Can you work these out from the model? Positions are in its coordinate system, mm. A direction names the side the tool comes from. Coordinates: 2 decimals unless noted, no trailing zeros. Order: outer loops, then holes, each group sorted by start corner. A loop starts at its lowest first (then second) coordinate and runs counter-clockwise, first axis right, second up. Notation, with made-up numbers: M 68.5,20 L 107.5,20 A8 cw 107.5,24 Z; hole C 69.5,79.25 d2. An arc over 180 degrees is marked long. Answer as CSV lines item,"result". Start each with the question number.
1. Will this pin go through, and if not, where does the flat tip stop? pin 1 (10 mm diameter, centred on x = 41, y = -49.5, fed in from -Z).
2. If we mould it in two halves opening along X, with no side actions, what happens to faces 3 (the face through (25, -61, 1.4)), 4 (the face through (-104.866, -60.837, 1.226)), 5 (the face through (-100.82, 56.74, 0.2)), 6 (the face through (100.82, -56.74, 0.2))? For each: released by +X, released by -X, zero draft, split by the parting line, or undercut.
3. I need wall thicknesses on line 1 along X through (y, z) = (-3, 0.4); line 2 along Y through (x, z) = (47.5, 0.45); line 3 along Y through (x, z) = (-3.5, 0.35). Which ranges of each line are inside material? Lowest first, please. Write a range as from..to.
4. If we section it at B-B (x = 53): List the corners of the cut face in (y, z) for me, plus the area to 3 significant figures.
5. On a 3-axis mill with a long thin cutter (end or side, diameter ignored), from which of +Z, -Z, +X, -X, +Y, -Y can I reach the whole of each face in a straight line? I mean faces 1 (the face through (-100.94, -56.62, 0.2)), 2 (the face through (-105.037, 60.666, 1.226)). Say none if no direction works.
6. If we section it at C-C (z = 0.65): List the corners of the cut face in (x, y) for me.
7. If we section it at A-A (y = -3.5): List the corners of the cut face in (x, z) for me.
```python
from build123d import *

# Parameters (mm, degrees)
PAD002_DEPTH = 1.4
FILLET_R     = 1
CHAMFER_SIZE = 1


with BuildPart() as part:
    # Sketch003 → Pad002 (new body)
    with BuildSketch(Plane.XY):
        with BuildLine():
            Line((-97.175786, 64.8), (97.175786, 64.8))
            ThreePointArc((109, 52.975786), (105.536768, 61.336768), (97.175786, 64.8))
            Line((109, 52.975786), (109, -52.975786))
            ThreePointArc((97.175786, -64.8), (105.536768, -61.336768), (109, -52.975786))
            Line((97.175786, -64.8), (-97.175786, -64.8))
            ThreePointArc((-109, -52.975786), (-105.536768, -61.336768), (-97.175786, -64.8))
            Line((-109, -52.975786), (-109, 52.975786))
            ThreePointArc((-97.175786, 64.8), (-105.536768, 61.336768), (-109, 52.975786))
        make_face()
        with BuildLine():
            Line((-95.761573, 58.8), (95.761573, 58.8))
            ThreePointArc((103, 51.561573), (100.879914, 56.679914), (95.761573, 58.8))
            Line((103, 51.561573), (103, -51.561573))
            ThreePointArc((95.761573, -58.8), (100.879914, -56.679914), (103, -51.561573))
            Line((95.761573, -58.8), (-95.761573, -58.8))
            ThreePointArc((-103, -51.561573), (-100.879914, -56.679914), (-95.761573, -58.8))
            Line((-103, -51.561573), (-103, 51.561573))
            ThreePointArc((-95.761573, 58.8), (-100.879914, 56.679914), (-103, 51.561573))
        make_face(mode=Mode.SUBTRACT)
    extrude(amount=PAD002_DEPTH)

    # Fillet
    fillet_edges = [part.edges().sort_by_distance(p)[0] for p in [
        (0, 58.8, 1.4),
        (-100.879914, 56.679914, 1.4),
        (-103, 0, 1.4),
        (-100.879914, -56.679914, 1.4),
        (0, -58.8, 1.4),
        (100.879914, -56.679914, 1.4),
        (103, 0, 1.4),
        (100.879914, 56.679914, 1.4),
    ]]
    fillet(fillet_edges, radius=FILLET_R)

    # Chamfer
    chamfer_edges = [part.edges().sort_by_distance(p)[0] for p in [
        (0, 64.8, 1.4),
        (105.536768, 61.336768, 1.4),
        (109, 0, 1.4),
        (105.536768, -61.336768, 1.4),
        (0, -64.8, 1.4),
        (-105.536768, -61.336768, 1.4),
        (-109, 0, 1.4),
        (-105.536768, 61.336768, 1.4),
    ]]
    chamfer(chamfer_edges, length=CHAMFER_SIZE)


solid = part.part
```
Solved:
1,pin 1,"through"
2,face 3,"zero draft"
2,face 4,"released by -X"
2,face 5,"undercut"
2,face 6,"undercut"
3,line 1,"-109..-103, 103..109"
3,line 2,"-64.75..-58.8, 58.8..64.75"
3,line 3,"-64.8..-58.8, 58.8..64.8"
4,outline,"M -64.8,0 L -58.8,0 L -58.8,0.4 A1 ccw -59.8,1.4 L -63.8,1.4 L -64.8,0.4 Z; M 58.8,0 L 64.8,0 L 64.8,0.4 L 63.8,1.4 L 59.8,1.4 A1 ccw 58.8,0.4 Z"
4,area,"15.4 mm²"
5,face 1,"+Z, -Z"
5,face 2,"+Z, -X, +Y"
6,outline,"M -108.75,-52.98 A11.57 ccw -97.18,-64.55 L 97.18,-64.55 A11.57 ccw 108.75,-52.98 L 108.75,52.98 A11.57 ccw 97.18,64.55 L -97.18,64.55 A11.57 ccw -108.75,52.98 Z; hole M -103.03,-51.56 A7.27 ccw -95.76,-58.83 L 95.76,-58.83 A7.27 ccw 103.03,-51.56 L 103.03,51.56 A7.27 ccw 95.76,58.83 L -95.76,58.83 A7.27 ccw -103.03,51.56 Z"
7,outline,"M -109,0 L -103,0 L -103,0.4 A1 ccw -104,1.4 L -108,1.4 L -109,0.4 Z; M 103,0 L 109,0 L 109,0.4 L 108,1.4 L 104,1.4 A1 ccw 103,0.4 Z"
